```python
from build123d import *

# Parameters (mm, degrees)
SKETCH1_W           = 30.988
SKETCH1_H           = 9.2075
BOSS_EXTRUDE1_DEPTH = 1.5875
SKETCH2_R           = 2.0066
BOSS_EXTRUDE2_DEPTH = 1.5875
FILLET1_R           = 12.7
FILLET2_R           = 5.08
CUT_EXTRUDE1_DEPTH  = 36.65115735


with BuildPart() as part:
    # Sketch1 → Boss-Extrude1 (new body)
    with BuildSketch(Plane.XY):
        with Locations((15.494, 4.60375)):
            Rectangle(SKETCH1_W, SKETCH1_H)
    extrude(amount=BOSS_EXTRUDE1_DEPTH)

    # Sketch2 → Boss-Extrude2 (add)
    with BuildSketch(Plane.XY.offset(1.5875)):
        with BuildLine():
            Line((15.588120411, 9.2075), (30.988, 9.2075))
            Line((30.988, 9.2075), (30.988, 16.312421236))
            ThreePointArc((30.988, 16.312421236), (25.682747304, 17.596645629), (20.843386501, 15.071665335))
            Line((20.843386501, 15.071665335), (15.588120411, 9.2075))
        make_face()
        with Locations((26.67, 13.742344032)):
            Circle(SKETCH2_R, mode=Mode.SUBTRACT)
    extrude(amount=-BOSS_EXTRUDE2_DEPTH)

    # Fillet1
    fillet1_edges = [part.edges().sort_by_distance(p)[0] for p in [
        (15.588120411, 9.2075, 0.79375),
    ]]
    fillet(fillet1_edges, radius=FILLET1_R)

    # Fillet2
    fillet2_edges = [part.edges().sort_by_distance(p)[0] for p in [
        (30.988, 16.312421236, 0.79375),
    ]]
    fillet(fillet2_edges, radius=FILLET2_R)

    # Sketch3 → Cut-Extrude1 (cut, through all)
    with BuildSketch(Plane.XY.offset(1.5875)):
        with BuildLine():
            Line((6.76275, 6.2865), (24.22525, 6.2865))
            ThreePointArc((24.22525, 6.2865), (25.908, 4.60375), (24.22525, 2.921))
            Line((24.22525, 2.921), (6.76275, 2.921))
            ThreePointArc((6.76275, 2.921), (5.08, 4.60375), (6.76275, 6.2865))
        make_face()
    extrude(amount=-CUT_EXTRUDE1_DEPTH, mode=Mode.SUBTRACT)


solid = part.part
```
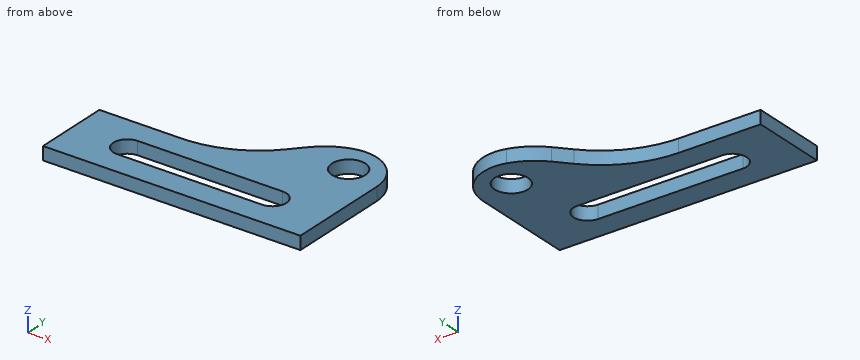
Source: CAD feature listing. Evaluate the final solid. Frame: model axes, mm. Round coordinates to 2 decimals unless told otherwise and drop trailing zeros. Loops run counter-clockwise (first coordinate to the right, second up) from the corner with the lowest first, then second, coordinate; pieces in that order, holes last.
1. Ray query, L1, parallel to Y at x = 25, z = 1.3; L2, parallel to X at y = 4, z = 0.8; L3, parallel to Y at x = 18, z = 1.2. Return the intervals inside material, ascending.
2. Section query C-C on z = 0.6. Output: boundary loops of the cut face in (x, y), and give its area (3 significant figures).
3. Section query B-B on y = 5. Output: boundary loops of the cut face in (x, z).
4. Section query A-A on x = 26.67. Output: boundary loops of the cut face in (y, z).
5. Contact query for a flat-ended pin moving along its axis: pin 1 (0.5 mm diameter, centred on x = 14, z = 1, fed in from +Y). Output: stop coordinate, or through.
Answers below:
1. L1: y = 0 to 3.11, 6.1 to 12.63, 14.85 to 17.47
1. L2: x = 0 to 5.19, 25.8 to 30.99
1. L3: y = 0 to 2.92, 6.29 to 12.11
2. outline: (0, 0) - (30.99, 0) - (30.99, 12.48) arc R5.08 ccw to (24.55, 17.37) arc R7.76 ccw to (20.84, 15.07) - (19.37, 13.43) arc R12.7 cw to (9.92, 9.21) - (0, 9.21) - close; hole (6.76, 2.92) - (24.23, 2.92) arc R1.68 ccw to (24.23, 6.29) - (6.76, 6.29) arc R1.68 ccw to start; hole circle Ø4.01 at (26.67, 13.74)
2. area: 300 mm2
3. outline: (0, 0) - (5.13, 0) - (5.13, 1.59) - (0, 1.59) - close; (25.86, 0) - (30.99, 0) - (30.99, 1.59) - (25.86, 1.59) - close
4. outline: (0, 0) - (11.74, 0) - (11.74, 1.59) - (0, 1.59) - close; (15.75, 0) - (17.5, 0) - (17.5, 1.59) - (15.75, 1.59) - close
5. pin 1: stops at y = 9.97
